```python
from build123d import *

# Parameters (mm, degrees)
BOSS_EXTRUDE1_DEPTH = 105
SKETCH2_R           = 8
BOSS_EXTRUDE2_DEPTH = 18
FILLET1_R           = 6
BOSS_EXTRUDE3_START = -20
BOSS_EXTRUDE3_DEPTH = 20


with BuildPart() as part:
    # Sketch1 → Boss-Extrude1 (new body)
    with BuildSketch(Plane.XY):
        Polygon((45, 0), (60, 0), (60, 25), (0, 25), (0, 0), (15, 0), (10, 14), (50, 14), align=None)
    extrude(amount=-BOSS_EXTRUDE1_DEPTH)

    # Sketch2 → Boss-Extrude2 (add)
    with BuildSketch(Plane.XY):
        with BuildLine():
            Line((15, 55), (15, 25))
            Line((15, 25), (45, 25))
            Line((45, 25), (45, 55))
            ThreePointArc((45, 55), (30, 70), (15, 55))
        make_face()
        with Locations((30, 55)):
            Circle(SKETCH2_R, mode=Mode.SUBTRACT)
    extrude(amount=-BOSS_EXTRUDE2_DEPTH)

    # Fillet1
    fillet1_edges = [part.edges().sort_by_distance(p)[0] for p in [
        (45, 25, -9),
        (15, 25, -9),
    ]]
    fillet(fillet1_edges, radius=FILLET1_R)

    # Sketch3 → Boss-Extrude3 (add)
    with BuildSketch(Plane(origin=(0, 0, -105), x_dir=(-1, 0, 0), z_dir=(0, 0, -1)).offset(BOSS_EXTRUDE3_START)):
        with BuildLine():
            Line((-60, 55), (-45, 70))
            Line((-45, 70), (-38, 70))
            Line((-38, 70), (-38, 55))
            ThreePointArc((-38, 55), (-30, 47), (-22, 55))
            Line((-22, 55), (-22, 70))
            Line((-22, 70), (-15, 70))
            Line((-15, 70), (0, 55))
            Line((0, 55), (0, 25))
            Line((0, 25), (-60, 25))
            Line((-60, 25), (-60, 55))
        make_face()
    extrude(amount=BOSS_EXTRUDE3_DEPTH)


solid = part.part
```
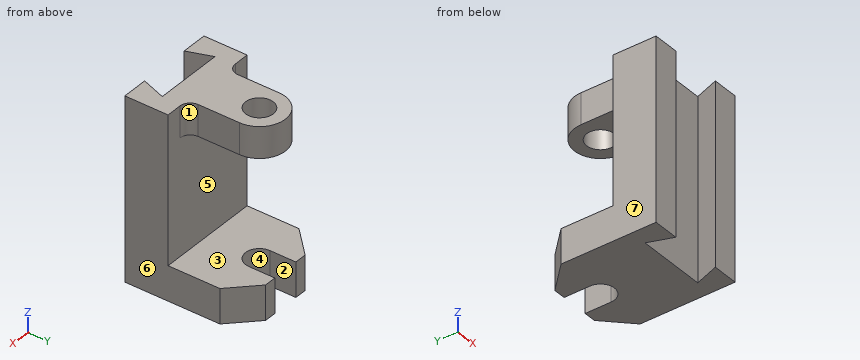
Model file for the job. Use its own axes, mm. Face numbers are marked on the shaded views. A direction names the side the tool comes from. Round coordinates to 2 decimals unless told otherwise and drop trailing zeros. Write each loop counter-clockwise with the first axis right and the second up, starting at its lowest first coordinate (ties: lowest second). Pieces come first, ordered by that corner, then holes. Notation, with made-up numbers: (13, 60.5) - (67, 60.5) arc R19 cw to (67, 81.5) - close; hole circle Ø5 at (43, 25). An arc over 180 degrees is marked (long way). One line per item, written item: value.
(1) Cut at D-D, the plane y = 61. Give the cut face in (x, z).
Values follow:
outline: (6, -105) - (22, -105) - (22, -85) - (6, -85) - close; (16.25, -18) - (24.71, -18) - (24.71, 0) - (16.25, 0) - close; (35.29, -18) - (43.75, -18) - (43.75, 0) - (35.29, 0) - close; (38, -105) - (54, -105) - (54, -85) - (38, -85) - close
(2) Wall check: probe 1 along Z at (x, y) = (40, 34); probe 2 along Y at (x, z) = (30, -5.5); probe 3 along Y at (x, z) = (36.5, -14). Give the ranges that are in metal, low to high.
Values follow:
probe 1: z = -105 to -85, -18 to 0
probe 2: y = 14 to 47, 63 to 70
probe 3: y = 14 to 50.34, 59.66 to 68.52
(3) Cut at C-C, the plane z = -46.5. Give the cut face in (x, y), plus the area to 3 significant figures.
Values follow:
outline: (0, 0) - (15, 0) - (10, 14) - (50, 14) - (45, 0) - (60, 0) - (60, 25) - (0, 25) - close
area: 1,010 mm²
(4) Cut at A-A, the plane y = 36. Give the cut face in (x, z), plus the area to 3 significant figures.
Values follow:
outline: (0, -105) - (60, -105) - (60, -85) - (0, -85) - close; (15, -18) - (45, -18) - (45, 0) - (15, 0) - close
area: 1,740 mm²
(5) 3-axis set-ups, long thin cutter, end or side, ignore diameter. For the marked faces 1, 2 and 3: which of +Z, -Z, +X, -X, +Y, -Y reach the whole face in a straight line?
Values follow:
face 1: +Z, +X, +Y
face 2: -Z, +Y
face 3: +X, -X, +Y
(6) Cut at B-B, the plane x = 30. Give the cut face in (y, z), plus the area to 3 significant figures.
Values follow:
outline: (14, -105) - (47, -105) - (47, -85) - (25, -85) - (25, -18) - (47, -18) - (47, 0) - (14, 0) - close; (63, -18) - (70, -18) - (70, 0) - (63, 0) - close
area: 2,120 mm²
(7) Drop flat-ended pins along their axis: P1, Ø14.5, axis at y = 44, z = -12.5, coming from the +X side; P2, Ø10, axis at y = 38, z = -24.5, coming from the +X side; P3, Ø14.5, axis at y = 46.5, z = -11.5, coming from the -X side. Give the stop position or say it passes through.
Values follow:
P1: stops at x = 45
P2: passes through
P3: stops at x = 15
(8) Two-plate mould, pull along X, no slides. Class the marked faces 4, 5, 6 and 7: pulls with the +X half, pulls with the -X half, needs draft (parallel to the pull), parting line crosses it, or undercut.
Values follow:
face 4: undercut
face 5: needs draft
face 6: pulls with the +X half
face 7: pulls with the -X half
